Design review of the part built by this model. Coordinates are the model's own, in mm. Round coordinates to 2 decimals unless told otherwise and drop trailing zeros. Write each loop counter-clockwise with the first axis right and the second up, starting at its lowest first coordinate (ties: lowest second). Pieces come first, ordered by that corner, then holes. Notation, with made-up numbers: (31.5, -4) - (53.5, -4) arc R35 ccw to (53.5, 35) - close; hole circle Ø7 at (2, 52.5). An arc over 180 degrees is marked (long way). Use one line per item in the form item = value.
```python
from build123d import *

# Parameters (mm, degrees)
F0_W     = 19.05
F0_H     = 19.05
F1_DEPTH = 3.175
F2_R     = 5.08


with BuildPart() as f1:
    # F0 (on Top) → F1 (new body, symmetric)
    with BuildSketch(Plane.XY):
        with Locations((-4.120239, 0)):
            Rectangle(F0_W, F0_H)
    extrude(amount=F1_DEPTH, both=True)

    # F2
    f2_edges = [f1.edges().sort_by_distance(p)[0] for p in [
        (-4.120239, -9.525, 3.175),
        (5.404761, 0, 3.175),
        (-4.120239, 9.525, 3.175),
        (-13.645239, 0, 3.175),
        (5.404761, -9.525, 0),
        (-13.645239, -9.525, 0),
        (-13.645239, 9.525, 0),
        (5.404761, 9.525, 0),
    ]]
    fillet(f2_edges, radius=F2_R)


solid = f1.part
```
Q1. We need section D-D on z = 1.5. Write out the cut boundary in (x, y) (3 decimals).
Calculated:
outline = (-12.335, -4.445) arc R3.77 ccw to (-8.565, -8.215) - (0.325, -8.215) arc R3.77 ccw to (4.095, -4.445) - (4.095, 4.445) arc R3.77 ccw to (0.325, 8.215) - (-8.565, 8.215) arc R3.77 ccw to (-12.335, 4.445) - close
Q2. To check wall thickness, follow line 1 along X through (y, z) = (1.75, -1.75); line 2 along X through (y, z) = (1.5, 2); line 3 along Z through (x, y) = (-9.5, -1.75) (3 decimals). State the ranges of each line that lie inside material, in increasing order. Write a range as from..to.
Calculated:
line_1 = -13.64..5.4
line_2 = -11.81..3.57
line_3 = -3.175..3.088
Q3. We need section B-B on z = -0.75. Write out the cut boundary in (x, y) (3 decimals), then the cut area to 3 significant figures.
Calculated:
outline = (-13.512, -4.445) arc R4.947 ccw to (-8.565, -9.392) - (0.325, -9.392) arc R4.947 ccw to (5.272, -4.445) - (5.272, 4.445) arc R4.947 ccw to (0.325, 9.392) - (-8.565, 9.392) arc R4.947 ccw to (-13.512, 4.445) - close
area = 332 mm2
Q4. For P1, Ø2, axis at x = -5, z = -1.5, coming from the -Y side (3 decimals); P2, Ø2, axis at y = 7.5, z = -1.5, coming from the +X side, all flat-tipped, find the tip position at first contact; note any pin that passes through.
Calculated:
P1 = -9.525
P2 = 4.96
Q5. We need section C-C on x = -5.75. Write out the cut boundary in (y, z) (3 decimals), then the cut area to 3 significant figures.
Calculated:
outline = (-9.525, -3.175) - (9.525, -3.175) - (9.525, -1.905) arc R5.08 ccw to (4.445, 3.175) - (-4.445, 3.175) arc R5.08 ccw to (-9.525, -1.905) - close
area = 110 mm2
Q6. We need section A-A on y = -2.25. Write out the cut boundary in (x, z) (3 decimals), then the cut area to 3 significant figures.
Calculated:
outline = (-13.645, -3.175) - (5.405, -3.175) - (5.405, -1.905) arc R5.08 ccw to (0.325, 3.175) - (-8.565, 3.175) arc R5.08 ccw to (-13.645, -1.905) - close
area = 110 mm2
